from build123d import *

# Parameters (mm, degrees)
CUT_EXTRUDE_1_DEPTH      = 69.82949949
CUT_EXTRUDE_1_DEPTH_BACK = 69.82949949
SKETCH_2_R               = 2
SKETCH_2_R_2             = 2.25
SKETCH_3_R               = 4
CUT_EXTRUDE_2_DEPTH      = 4.4
FILLET_1_R               = 1


with BuildPart() as part:
    # 草图1 → 旋转1 (revolve)
    with BuildSketch(Plane.XY, mode=Mode.PRIVATE) as revolve_1_sk:
        Polygon((17.5, 7.5), (17.5, -7.5), (29.5, -7.5), (29.5, -5.5), (35.5, -5.5), (35.5, -7.5), (47.5, -7.5), (47.5, 7.5), (35.5, 7.5), (35.5, 5.5), (29.5, 5.5), (29.5, 7.5), align=None)
    revolve(revolve_1_sk.sketch.rotate(Axis((0, 50.744480159, 0), (0, -1, 0)), 90), axis=Axis((0, 50.744480159, 0), (0, -1, 0)))

    # 草图2 → 切除-拉伸1 (cut, two sides: drawn at the far end of the back side and taken through both)
    with BuildSketch(Plane(origin=(0, 7.5, 0), x_dir=(1, 0, 0), z_dir=(0, 1, 0)).offset(-CUT_EXTRUDE_1_DEPTH_BACK)):
        with Locations(Location((0, 22.5, 0), (0, 0, 270))):
            Circle(SKETCH_2_R)
        with Locations(Location((0, 41.5, 0), (0, 0, 270))):
            Circle(SKETCH_2_R_2)
        with Locations(Location((15.909902577, 15.909902577, 0), (0, 0, 270))):
            Circle(SKETCH_2_R)
        with Locations(Location((22.5, 0, 0), (0, 0, 270))):
            Circle(SKETCH_2_R)
        with Locations(Location((15.909902577, -15.909902577, 0), (0, 0, 270))):
            Circle(SKETCH_2_R)
        with Locations(Location((0, -22.5, 0), (0, 0, 270))):
            Circle(SKETCH_2_R)
        with Locations(Location((-15.909902577, -15.909902577, 0), (0, 0, 270))):
            Circle(SKETCH_2_R)
        with Locations(Location((-22.5, 0, 0), (0, 0, 270))):
            Circle(SKETCH_2_R)
        with Locations(Location((-15.909902577, 15.909902577, 0), (0, 0, 270))):
            Circle(SKETCH_2_R)
        with Locations(Location((29.344931419, 29.344931419, 0), (0, 0, 270))):
            Circle(SKETCH_2_R_2)
        with Locations(Location((41.5, 0, 0), (0, 0, 270))):
            Circle(SKETCH_2_R_2)
        with Locations(Location((29.344931419, -29.344931419, 0), (0, 0, 270))):
            Circle(SKETCH_2_R_2)
        with Locations(Location((0, -41.5, 0), (0, 0, 270))):
            Circle(SKETCH_2_R_2)
        with Locations(Location((-29.344931419, -29.344931419, 0), (0, 0, 270))):
            Circle(SKETCH_2_R_2)
        with Locations(Location((-41.5, 0, 0), (0, 0, 270))):
            Circle(SKETCH_2_R_2)
        with Locations(Location((-29.344931419, 29.344931419, 0), (0, 0, 270))):
            Circle(SKETCH_2_R_2)
    extrude(amount=CUT_EXTRUDE_1_DEPTH + CUT_EXTRUDE_1_DEPTH_BACK, mode=Mode.SUBTRACT)

    # 草图3 → 切除-拉伸2 (cut)
    with BuildSketch(Plane(origin=(0, 7.5, 0), x_dir=(1, 0, 0), z_dir=(0, 1, 0))):
        with Locations(Location((0, 41.5, 0), (0, 0, 270))):
            Circle(SKETCH_3_R)
        with Locations(Location((29.344931419, 29.344931419, 0), (0, 0, 270))):
            Circle(SKETCH_3_R)
        with Locations(Location((41.5, 0, 0), (0, 0, 270))):
            Circle(SKETCH_3_R)
        with Locations(Location((29.344931419, -29.344931419, 0), (0, 0, 270))):
            Circle(SKETCH_3_R)
        with Locations(Location((0, -41.5, 0), (0, 0, 270))):
            Circle(SKETCH_3_R)
        with Locations(Location((-29.344931419, -29.344931419, 0), (0, 0, 270))):
            Circle(SKETCH_3_R)
        with Locations(Location((-41.5, 0, 0), (0, 0, 270))):
            Circle(SKETCH_3_R)
        with Locations(Location((-29.344931419, 29.344931419, 0), (0, 0, 270))):
            Circle(SKETCH_3_R)
    extrude(amount=-CUT_EXTRUDE_2_DEPTH, mode=Mode.SUBTRACT)

    # 圆角1
    fillet_1_edges = [part.edges().sort_by_distance(p)[0] for p in [
        (0, -7.5, -47.5),
        (0, 7.5, -47.5),
        (0, 7.5, -17.5),
        (0, -7.5, -17.5),
    ]]
    fillet(fillet_1_edges, radius=FILLET_1_R)


solid = part.part
Geometry check sheet. Reference: the model listing, model coordinates, mm. A direction names the side the tool comes from. Coordinates: 2 decimals unless noted, no trailing zeros. Use one line per item in the form item = value. Start each with the question number.
Item 1: Tool access check on faces 3 (the face through (34.656, -6.514, -7.696)), 4 (the face through (-37.534, 5.331, -0.521)), 5 (the face through (-31.2, 7.5, -17.4)). Record the directions out of +Z, -Z, +X, -X, +Y, -Y that give a thin tool (end or side, any length) a straight path to the whole face; none if there is none.
Item 2: Mould release check, pull along X, two halves, no side actions. Record for faces 1 (the face through (-14, -7.5, -13)), 2 (the face through (16.511, -0.105, 17.818)): +X half, -X half, draft (parallel to the pull), parting line (faces both ways), or undercut.
Item 3: Gauge pin test, flat ends, axial feed: pin 1 (6 mm diameter, centred on x = 0, z = -41.5, fed in from +Y); pin 2 (1.5 mm diameter, centred on x = -11.5, y = -5.5, fed in from -Z); pin 3 (2 mm diameter, centred on y = 1, z = -37, fed in from +X). Record the tip position at first contact, or that the pin passes through.
Item 4: Thickness scan on probe 1 along Z at (x, y) = (-30.5, 0); probe 2 along X at (y, z) = (0.75, 0); probe 3 along Z at (x, y) = (-31, 4). Record the ranges inside material, lowest first.
Item 5: Section check A-A, the plane y = -2.5. Give the number of separate pieces and of enclosed holes in the cut face, and give its area (3 significant figures).
Computed:
q1.face_3 = -Y
q1.face_4 = +Y
q1.face_5 = +Z, -Z, +X, -X, +Y
q2.face_1 = draft
q2.face_2 = undercut
q3.pin_1 = 3.1
q3.pin_2 = -46.27
q3.pin_3 = 30.99
q4.probe_1 = -36.41 to -31.28, -27.41 to 27.41, 31.28 to 36.41
q4.probe_2 = -47.5 to -43.75, -39.25 to -24.5, -20.5 to -17.5, 17.5 to 20.5, 24.5 to 39.25, 43.75 to 47.5
q4.probe_3 = -35.99 to -32.99, -25.7 to 25.7, 32.99 to 35.99
q5.separate_pieces = 1
q5.enclosed_holes = 17
q5.area = 5,900 mm2
